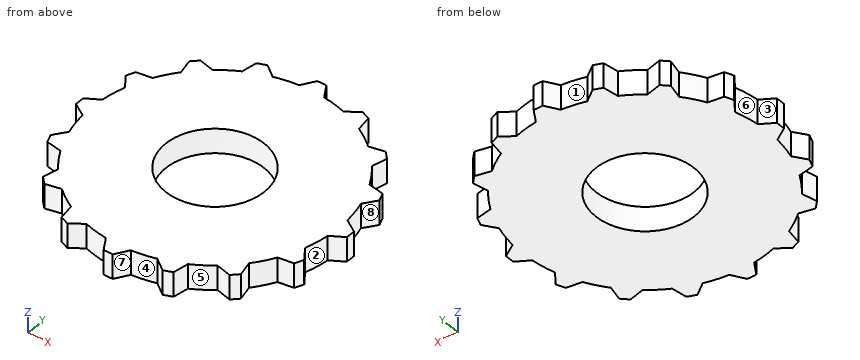
```python
from build123d import *

# Parameters (mm, degrees)
SKETCH1_R           = 20
BOSS_EXTRUDE1_DEPTH = 10


with BuildPart() as part:
    # Sketch1 → Boss-Extrude1 (new body)
    with BuildSketch(Plane.XY):
        with BuildLine():
            Line((1.826311743, 54.969669686), (-1.826311743, 54.969669686))
            Line((-1.826311743, 54.969669686), (-5.055544828, 49.743758066))
            ThreePointArc((-5.055544828, 49.743758066), (-9.754516101, 49.03926402), (-14.365397683, 47.891913194))
            Line((-14.365397683, 47.891913194), (-19.348689832, 51.484251979))
            Line((-19.348689832, 51.484251979), (-22.723273911, 50.086453485))
            Line((-22.723273911, 50.086453485), (-23.706826468, 44.0225667))
            ThreePointArc((-23.706826468, 44.0225667), (-27.778511651, 41.573480615), (-31.599338619, 38.74895868))
            Line((-31.599338619, 38.74895868), (-37.578028776, 40.160823613))
            Line((-37.578028776, 40.160823613), (-40.160823613, 37.578028776))
            Line((-40.160823613, 37.578028776), (-38.74895868, 31.599338619))
            ThreePointArc((-38.74895868, 31.599338619), (-41.573480615, 27.778511651), (-44.0225667, 23.706826468))
            Line((-44.0225667, 23.706826468), (-50.086453485, 22.723273911))
            Line((-50.086453485, 22.723273911), (-51.484251979, 19.348689832))
            Line((-51.484251979, 19.348689832), (-47.891913194, 14.365397683))
            ThreePointArc((-47.891913194, 14.365397683), (-49.03926402, 9.754516101), (-49.743758066, 5.055544828))
            Line((-49.743758066, 5.055544828), (-54.969669686, 1.826311743))
            Line((-54.969669686, 1.826311743), (-54.969669686, -1.826311743))
            Line((-54.969669686, -1.826311743), (-49.743758066, -5.055544828))
            ThreePointArc((-49.743758066, -5.055544828), (-49.03926402, -9.754516101), (-47.891913194, -14.365397683))
            Line((-47.891913194, -14.365397683), (-51.484251979, -19.348689832))
            Line((-51.484251979, -19.348689832), (-50.086453485, -22.723273911))
            Line((-50.086453485, -22.723273911), (-44.0225667, -23.706826468))
            ThreePointArc((-44.0225667, -23.706826468), (-41.573480615, -27.778511651), (-38.74895868, -31.599338619))
            Line((-38.74895868, -31.599338619), (-40.160823613, -37.578028776))
            Line((-40.160823613, -37.578028776), (-37.578028776, -40.160823613))
            Line((-37.578028776, -40.160823613), (-31.599338619, -38.74895868))
            ThreePointArc((-31.599338619, -38.74895868), (-27.778511651, -41.573480615), (-23.706826468, -44.0225667))
            Line((-23.706826468, -44.0225667), (-22.723273911, -50.086453485))
            Line((-22.723273911, -50.086453485), (-19.348689832, -51.484251979))
            Line((-19.348689832, -51.484251979), (-14.365397683, -47.891913194))
            ThreePointArc((-14.365397683, -47.891913194), (-9.754516101, -49.03926402), (-5.055544828, -49.743758066))
            Line((-5.055544828, -49.743758066), (-1.826311743, -54.969669686))
            Line((-1.826311743, -54.969669686), (1.826311743, -54.969669686))
            Line((1.826311743, -54.969669686), (5.055544828, -49.743758066))
            ThreePointArc((5.055544828, -49.743758066), (9.754516101, -49.03926402), (14.365397683, -47.891913194))
            Line((14.365397683, -47.891913194), (19.348689832, -51.484251979))
            Line((19.348689832, -51.484251979), (22.723273911, -50.086453485))
            Line((22.723273911, -50.086453485), (23.706826468, -44.0225667))
            ThreePointArc((23.706826468, -44.0225667), (27.778511651, -41.573480615), (31.599338619, -38.74895868))
            Line((31.599338619, -38.74895868), (37.578028776, -40.160823613))
            Line((37.578028776, -40.160823613), (40.160823613, -37.578028776))
            Line((40.160823613, -37.578028776), (38.74895868, -31.599338619))
            ThreePointArc((38.74895868, -31.599338619), (41.573480615, -27.778511651), (44.0225667, -23.706826468))
            Line((44.0225667, -23.706826468), (50.086453485, -22.723273911))
            Line((50.086453485, -22.723273911), (51.484251979, -19.348689832))
            Line((51.484251979, -19.348689832), (47.891913194, -14.365397683))
            ThreePointArc((47.891913194, -14.365397683), (49.03926402, -9.754516101), (49.743758066, -5.055544828))
            Line((49.743758066, -5.055544828), (54.969669686, -1.826311743))
            Line((54.969669686, -1.826311743), (54.969669686, 1.826311743))
            Line((54.969669686, 1.826311743), (49.743758066, 5.055544828))
            ThreePointArc((49.743758066, 5.055544828), (49.03926402, 9.754516101), (47.891913194, 14.365397683))
            Line((47.891913194, 14.365397683), (51.484251979, 19.348689832))
            Line((51.484251979, 19.348689832), (50.086453485, 22.723273911))
            Line((50.086453485, 22.723273911), (44.0225667, 23.706826468))
            ThreePointArc((44.0225667, 23.706826468), (41.573480615, 27.778511651), (38.74895868, 31.599338619))
            Line((38.74895868, 31.599338619), (40.160823613, 37.578028776))
            Line((40.160823613, 37.578028776), (37.578028776, 40.160823613))
            Line((37.578028776, 40.160823613), (31.599338619, 38.74895868))
            ThreePointArc((31.599338619, 38.74895868), (27.778511651, 41.573480615), (23.706826468, 44.0225667))
            Line((23.706826468, 44.0225667), (22.723273911, 50.086453485))
            Line((22.723273911, 50.086453485), (19.348689832, 51.484251979))
            Line((19.348689832, 51.484251979), (14.365397683, 47.891913194))
            ThreePointArc((14.365397683, 47.891913194), (9.754516101, 49.03926402), (5.055544828, 49.743758066))
            Line((5.055544828, 49.743758066), (1.826311743, 54.969669686))
        make_face()
        Circle(SKETCH1_R, mode=Mode.SUBTRACT)
    extrude(amount=BOSS_EXTRUDE1_DEPTH)


solid = part.part
```
Geometry check sheet. Reference: the model listing, model coordinates, mm. Face numbers are marked on the shaded views. A direction names the side the tool comes from. Coordinates: 2 decimals unless noted, no trailing zeros. Order: outer loops, then holes, each group sorted by start corner. A loop starts at its lowest first (then second) coordinate and runs counter-clockwise, first axis right, second up. Notation, with made-up numbers: (43.25, -4) - (99.25, -4) arc R24 ccw to (99.25, 35) - close; hole circle Ø5 at (38, -35). An arc over 180 degrees is marked (long way). Answer as a JSON object with one key per item and string values. Group by question number.
Item 1: Sectioned sample at C-C, the plane y = -46.5. Record the cut outline in (x, z) (3 decimals), and give its area (3 significant figures).
Item 2: Sectioned sample at A-A, the plane x = 0. Record the cut outline in (y, z), and give its area (3 significant figures).
Item 3: Tool access check on the marked faces 1, 2, 3 and 4. Record the directions out of +Z, -Z, +X, -X, +Y, -Y that give a thin tool (end or side, any length) a straight path to the whole face; none if there is none.
Item 4: Sectioned sample at D-D, the plane y = 29. Record the cut outline in (x, z), and give its area (3 significant figures).
Item 5: Depth check by flat-ended pin: pin 1 Ø2 at (x, z) = (-22, 1.5) entering from +Y; pin 2 Ø3 at (y, z) = (-27, 6.5) entering from +X; pin 3 Ø6 at (y, z) = (-11, 3) entering from -X; pin 4 Ø10 at (x, y) = (7.5, -8) entering from +Z. Enter the tip coordinate at first touch or a pass-through.
Item 6: Scan lines: probe 1 along Y at (x, z) = (0, 2.25); probe 2 along Y at (x, z) = (50.5, 8.75); probe 3 along Y at (x, z) = (-10.5, 4.25). Record each from-to range of solid material in increasing order.
Item 7: Draft check along X on the marked faces 5, 6, 7 and 8. Enter one of: +X half, -X half, draft (parallel to the pull), parting line (faces both ways), or undercut.
Resolved:
{
 "1": {"outline": "(-23.305, 0) - (23.305, 0) - (23.305, 10) - (-23.305, 10) - close", "area": "466 mm^2"},
 "2": {"outline": "(-54.97, 0) - (-20, 0) - (-20, 10) - (-54.97, 10) - close; (20, 0) - (54.97, 0) - (54.97, 10) - (20, 10) - close", "area": "699 mm^2"},
 "3": {"face 1": "+Z, -Z, +Y", "face 2": "+Z, -Z, +X", "face 3": "+Z, -Z, -X", "face 4": "+Z, -Z, -Y"},
 "4": {"outline": "(-40.73, 0) - (40.73, 0) - (40.73, 10) - (-40.73, 10) - close", "area": "815 mm^2"},
 "5": {"pin 1": "y = 50.8", "pin 2": "x = 43.01", "pin 3": "x = -49.36", "pin 4": "through"},
 "6": {"probe 1": "-54.97 to -20, 20 to 54.97", "probe 2": "-21.72 to -17.98, -4.59 to 4.59, 17.98 to 21.72", "probe 3": "-48.89 to -17.02, 17.02 to 48.89"},
 "7": {"face 5": "undercut", "face 6": "-X half", "face 7": "undercut", "face 8": "+X half"}
}
